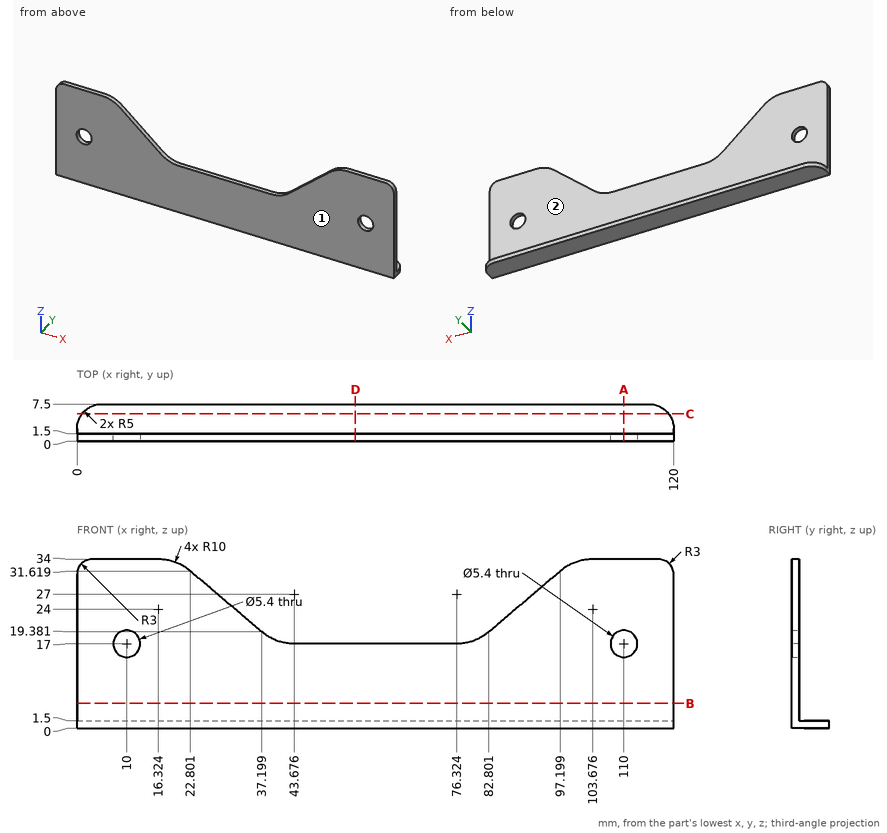
Check sheet for the drawn part. Datum: minimum x, y, z corner. Units: mm. A direction names the side the tool comes from. Give positions to 0.01 mm unless a question says otherwise; leave off trailing zeros. Write each loop counter-clockwise with the first axis right and the second up, starting at its lowest first coordinate (ties: lowest second). Pieces come first, ordered by that corner, then holes. Notation, with made-up numbers: (82.5, 68) -> (122.5, 68) arc R15 ccw to (122.5, 96) -> close; hole circle Ø7 at (53, 63.25). An arc over 180 degrees is marked (long way). Use one line per item in the form item = value. Start each with the question number.
1. Access from +Z, -Z, +X, -X, +Y, -Y to the whole of each face (thin tool, end or side, straight path). Record for the marked faces 1 and 2.
2. Thickness scan on line 1 along Z through (x, y) = (110, 0.9); line 2 along Z through (x, y) = (63.5, 4.5). Record the ranges inside material, lowest first. Write a range as from..to.
3. Go/stop test with flat-tipped pins: P1, Ø1.5, axis at x = 18.5, z = 11, coming from the -Y side; P2, Ø1.2, axis at x = 56, y = 0.5, coming from the +Z side; P3, Ø8.5, axis at x = 10, z = 17, coming from the +Y side; P4, Ø1.8, axis at x = 70.5, y = 3.5, coming from the +Z side. Record where each tip stops, or that it passes through.
4. Section check A-A (x = 110). Record the cut outline in (y, z).
5. Section check C-C (y = 5.5). Record the cut outline in (x, z), and give its area (3 significant figures).
6. Section check B-B (z = 5). Record the cut outline in (x, y).
7. Section check D-D (x = 56). Record the cut outline in (y, z).
Conclusion:
q1.face_1 = +Z, -Z, +X, -X, -Y
q1.face_2 = +Z, +X, -X, +Y
q2.line_1 = 0..14.3, 19.7..34
q2.line_2 = 0..1.5
q3.P1 = 0
q3.P2 = 17
q3.P3 = 1.5
q3.P4 = 1.5
q4.outline = (0, 0) -> (7.5, 0) -> (7.5, 1.5) -> (1.5, 1.5) -> (1.5, 14.3) -> (0, 14.3) -> close; (0, 19.7) -> (1.5, 19.7) -> (1.5, 34) -> (0, 34) -> close
q5.outline = (1, 0) -> (119, 0) -> (119, 1.5) -> (1, 1.5) -> close
q5.area = 177 mm²
q6.outline = (0, 0) -> (120, 0) -> (120, 1.5) -> (0, 1.5) -> close
q7.outline = (0, 0) -> (7.5, 0) -> (7.5, 1.5) -> (1.5, 1.5) -> (1.5, 17) -> (0, 17) -> close
